Could you check a few things on this model? Use its own coordinates, in mm. Face numbers are marked on the shaded views. A direction names the side the tool comes from. Round coordinates to 2 decimals unless told otherwise and drop trailing zeros. Loops run counter-clockwise (first coordinate to the right, second up) from the corner with the lowest first, then second, coordinate; pieces in that order, holes last. Notation, with made-up numbers: (86, 38.25) -> (135, 38.25) arc R16 cw to (135, 58.25) -> close; hole circle Ø11 at (-20.75, 84). An arc over 180 degrees is marked (long way). One line per item, written item: value.
Autodesk Inventor part; units mm, degrees
ref_plane "YZ Plane" through (0, 0, 0) normal (1, 0, 0) x (0, 1, 0)
ref_plane "XZ Plane" through (0, 0, 0) normal (0, 1, 0) x (-1, 0, 0)
ref_plane "XY Plane" through (0, 0, 0) normal (0, 0, 1) x (1, 0, 0)
sketch "Sketch1" plane through (0, 0, 0) normal (0, 1, 0) x (-1, 0, 0)
  line L0 (-9.5, -3) -> (6.5, -3)
  line L1 (6.5, -3) -> (6.5, 3)
  line L2 (6.5, 3) -> (-9.5, 3)
  line L3 (-9.5, 3) -> (-9.5, -3)
  circle A0 centre (3.5, 0) radius 2
  circle A1 centre (-3.5, 0) radius 2
  point P0 (0, 0)
  dimension "d0" = 4
  dimension "d3" = 3.5
  dimension "d4" = 4
  dimension "d5" = 3.5
  dimension "d6" = 7
  dimension "d7" = 6
  dimension "d8" = 3
  dimension "d9" = 3
  dimension "d10" = 3
  dimension "d11" = 6
extrude "Bottom Extrusion" add sketch "Sketch1" along normal blind 3
sketch "Sketch2" plane through (0, 3, 0) normal (0, 1, 0) x (1, 0, 0)
  line L0 (-6.5, -3) -> (9.5, -3) construction
  line L1 (9.5, -3) -> (9.5, 3) construction
  line L2 (9.5, 3) -> (6.5, 3)
  line L3 (6.5, 3) -> (6.5, -3)
  line L4 (6.5, -3) -> (9.5, -3)
  line L5 (9.5, -3) -> (9.5, 3)
  point P0 (0, 0)
  dimension "d14" = 3
extrude "Top Extrusion" add sketch "Sketch2" along normal blind 16
sketch "Sketch3" plane through (9.5, 0, 3) normal (1, 0, 0) x (0, 0, -1)
  line L0 (0, 19) -> (6, 19) construction
  circle A0 centre (3, 5) radius 2
  circle A1 centre (3, 15) radius 2
  point P0 (3, 0)
  dimension "d17" = 4
  dimension "d18" = 5
  dimension "d19" = 4
  dimension "d20" = 10
  dimension "d21" = 4
extrude "Top Holes" cut sketch "Sketch3" against normal through all
properties part number "Servo Locks V3"
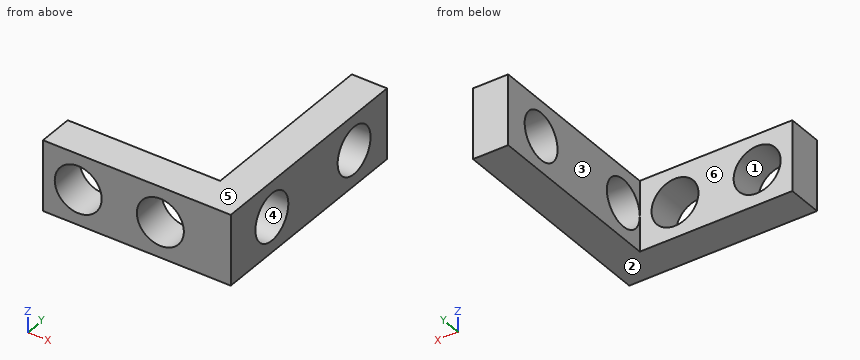
(1) If we section it at C-C, the plane z = -0.6: Please give me the cut outline in (x, y).
Recorded:
outline: (-6.5, 0) -> (-5.41, 0) -> (-5.41, 3) -> (-6.5, 3) -> close; (-1.59, 0) -> (1.59, 0) -> (1.59, 3) -> (-1.59, 3) -> close; (5.41, 0) -> (9.5, 0) -> (9.5, 3.09) -> (6.5, 3.09) -> (6.5, 3) -> (5.41, 3) -> close; (6.5, 6.91) -> (9.5, 6.91) -> (9.5, 13.09) -> (6.5, 13.09) -> close; (6.5, 16.91) -> (9.5, 16.91) -> (9.5, 19) -> (6.5, 19) -> close
(2) Thinking about a two-plate mould opening in Z: for the marked faces 1, 2, 3 and 4, which applies, released by +Z, released by -Z, zero draft, split by the parting line, or undercut?
Recorded:
face 1: undercut
face 2: released by -Z
face 3: zero draft
face 4: undercut
(3) If we section it at D-D, the plane x = -1.25: Please give me the cut outline in (y, z), then the cut area to 3 significant figures.
Recorded:
outline: (0, -3) -> (3, -3) -> (3, 3) -> (0, 3) -> close
area: 18.0 mm²
(4) If I drill on L1, parallel to X at y = 2.2, z = 0; L2, parallel to Y at x = 8.5, z = 0.1; L3, parallel to Z at x = 8.1, y = 5, over which ranges is the centre line in solid material (lowest first)?
Recorded:
L1: -6.5 to -5.5, -1.5 to 1.5, 5.5 to 9.5
L2: 0 to 3, 7 to 13, 17 to 19
L3: -3 to -2, 2 to 3
(5) For the marked faces 5 and 6, which set-ups out of +Z, -Z, +X, -X, +Y, -Y let a thin tool reach every point of the face, with its end or its side?
Recorded:
face 5: +Z, +X, -X, +Y, -Y
face 6: +Z, -Z, -X, +Y
(6) I'm going to push flat-ended pins straight in: pin 1 Ø1.8 at (y, z) = (7.5, 1.5) entering from -X; pin 2 Ø3 at (y, z) = (5, 0) entering from -X (1 decimal); pin 3 Ø1.5 at (x, z) = (-2, 1) entering from +Y. Where does each tip first touch, or does it pass through?
Recorded:
pin 1: x = 6.5
pin 2: through
pin 3: y = 3
(7) If we section it at B-B, the plane y = 5: Please give me the cut outline in (x, z).
Recorded:
outline: (6.5, -3) -> (9.5, -3) -> (9.5, -2) -> (6.5, -2) -> close; (6.5, 2) -> (9.5, 2) -> (9.5, 3) -> (6.5, 3) -> close
(8) If we section it at A-A, the plane x = -3.5: Please give me the cut outline in (y, z).
Recorded:
outline: (0, -3) -> (3, -3) -> (3, -2) -> (0, -2) -> close; (0, 2) -> (3, 2) -> (3, 3) -> (0, 3) -> close
